Source: CAD feature listing. Evaluate the final solid. Frame: model axes, mm. Face numbers are marked on the shaded views. A direction names the side the tool comes from. Give positions to 0.01 mm unless a question says otherwise; leave off trailing zeros. Loops run counter-clockwise (first coordinate to the right, second up) from the corner with the lowest first, then second, coordinate; pieces in that order, holes last. Notation, with made-up numbers: M 21,86.5 L 46,86.5 A22 ccw 46,93.5 Z; hole C 29.5,25.25 d9. An arc over 180 degrees is marked long. Put each result on its own line as item: value. Start each with the question number.
```python
from build123d import *

# Parameters (mm, degrees)
SKETCH_1_R          = 17.5
SKETCH_1_R_2        = 1.75
EXTRUDE_1_DEPTH     = 5
SKETCH_2_R          = 3
CUT_EXTRUDE_1_DEPTH = 3
SKETCH_3_R          = 10
SKETCH_6_R          = 6


with BuildPart() as part:
    # 草图1 → 凸台-拉伸1 (new body)
    with BuildSketch(Plane(origin=(0, 0, 0), x_dir=(1, 0, 0), z_dir=(0, 1, 0))):
        Circle(SKETCH_1_R)
        with Locations((0, 13.5)):
            Circle(SKETCH_1_R_2, mode=Mode.SUBTRACT)
        with Locations((11.691342951, 6.75)):
            Circle(SKETCH_1_R_2, mode=Mode.SUBTRACT)
        with Locations((11.691342951, -6.75)):
            Circle(SKETCH_1_R_2, mode=Mode.SUBTRACT)
        with Locations((0, -13.5)):
            Circle(SKETCH_1_R_2, mode=Mode.SUBTRACT)
        with Locations((-11.691342951, -6.75)):
            Circle(SKETCH_1_R_2, mode=Mode.SUBTRACT)
        with Locations((-11.691342951, 6.75)):
            Circle(SKETCH_1_R_2, mode=Mode.SUBTRACT)
    extrude(amount=EXTRUDE_1_DEPTH)

    # 草图2 → 切除-拉伸1 (cut)
    with BuildSketch(Plane(origin=(0, 5, 0), x_dir=(1, 0, 0), z_dir=(0, 1, 0))):
        with Locations((0, 13.5)):
            Circle(SKETCH_2_R)
        with Locations((11.691342951, 6.75)):
            Circle(SKETCH_2_R)
        with Locations((11.691342951, -6.75)):
            Circle(SKETCH_2_R)
        with Locations((0, -13.5)):
            Circle(SKETCH_2_R)
        with Locations((-11.691342951, -6.75)):
            Circle(SKETCH_2_R)
        with Locations((-11.691342951, 6.75)):
            Circle(SKETCH_2_R)
    extrude(amount=-CUT_EXTRUDE_1_DEPTH, mode=Mode.SUBTRACT)

    # 草图3 → 放样1 section 0
    with BuildSketch(Plane(origin=(0, 5, 0), x_dir=(1, 0, 0), z_dir=(0, 1, 0))):
        Circle(SKETCH_3_R)
    # 草图6 → 放样1 section 1
    with BuildSketch(Plane(origin=(0, 72, 0), x_dir=(1, 0, 0), z_dir=(0, 1, 0))):
        Circle(SKETCH_6_R)
    loft()

    # 草图7 → 旋转7 (revolve)
    with BuildSketch(Plane(origin=(0, 72, 0), x_dir=(1, 0, 0), z_dir=(0, 1, 0))):
        with BuildLine():
            Line((-8, 0), (8, 0))
            ThreePointArc((8, 0), (0, 8), (-8, 0))
        make_face()
    revolve(axis=Axis((-8, 72, 0), (1, 0, 0)))


solid = part.part
```
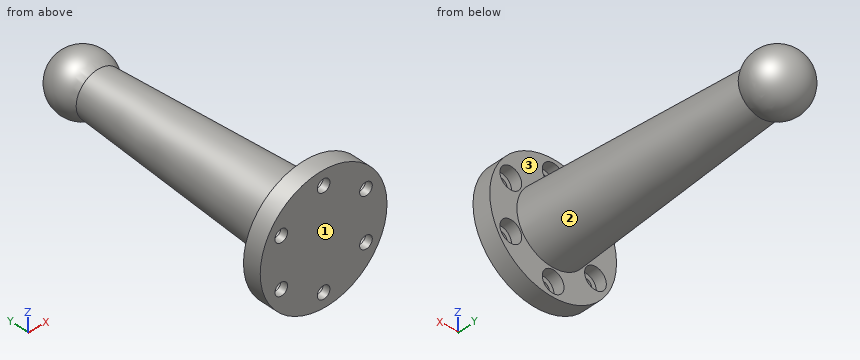
1. Set-up query: the marked faces 1, 2 and 3. Return all of +Z, -Z, +X, -X, +Y, -Y with unobstructed straight access to the full face (end or side cutting, diameter ignored); none if empty.
2. Section C-C, the plane y = 49. Output: boundary loops of the cut face in (x, z).
3. Section D-D, the plane z = 6.75. State how many separate pieces and enclosed holes the cut face has, plus the area to 3 significant figures.
4. Section B-B, the plane x = 0. Output: boundary loops of the cut face in (y, z).
5. Section A-A, the plane z = 13.5. Output: boundary loops of the cut face in (x, y), plus the area to 3 significant figures.
6. Contact query for flat-ended pins moving along their axis: pin 1 (12 mm diameter, centred on x = -3.5, z = 11.5, fed in from +Y); pin 2 (10 mm diameter, centred on x = -8, y = 51, fed in from +Z); pin 3 (8 mm diameter, centred on x = -9, y = 15.5, fed in from -Z). Output: stop coordinate, or through.
7. Ray query, line 1 (Z direction, x = 0, y = 1); line 2 (X direction, y = 0.65, z = -6.75); line 3 (Y direction, x = 1, z = 16). Return the intervals inside material, ascending.
Results found:
1. face 1: +Z, -Z, +X, -X, -Y
1. face 2: none
1. face 3: +Y
2. outline: C 0,0 d14.75
3. separate pieces: 4
3. enclosed holes: 0
3. area: 684 mm²
4. outline: M 0,-17.5 L 5,-17.5 L 5,-16.5 L 2,-16.5 L 2,-15.25 L 0,-15.25 Z; M 0,-11.75 L 2,-11.75 L 2,-10.5 L 5,-10.5 L 5,-10 L 67.06,-6.29 A8 ccw long 67.06,6.29 L 5,10 L 5,10.5 L 2,10.5 L 2,11.75 L 0,11.75 Z; M 0,15.25 L 2,15.25 L 2,16.5 L 5,16.5 L 5,17.5 L 0,17.5 Z
5. outline: M -11.14,0 L -1.75,0 L -1.75,2 L -3,2 L -3,5 L -11.14,5 Z; M 1.75,0 L 11.14,0 L 11.14,5 L 3,5 L 3,2 L 1.75,2 Z
5. area: 86.4 mm²
6. pin 1: y = 77.27
6. pin 2: z = 6.63
6. pin 3: z = -7.94
7. line 1: -17.5 to -15.25, -11.75 to 11.75, 15.25 to 17.5
7. line 2: -16.15 to -13.44, -9.94 to 9.94, 13.44 to 16.15
7. line 3: 0 to 2
